```python
from build123d import *

# Parameters (mm, degrees)
CROQUIS1_W              = 15
CROQUIS1_H              = 12
SALIENTE_EXTRUIR1_DEPTH = 2
CORTAR_EXTRUIR1_REACH   = 11.811
CROQUIS2_R              = 2
CROQUIS3_W              = 33
CROQUIS3_H              = 17
SALIENTE_EXTRUIR2_DEPTH = 2
CORTAR_EXTRUIR3_REACH   = 26.192
CROQUIS5_W              = 8
CROQUIS5_H              = 3
CORTAR_EXTRUIR4_REACH   = 27.244
CROQUIS6_R              = 2
REDONDEO1_R             = 3
REDONDEO2_R             = 3


with BuildPart() as part:
    # Croquis1 → Saliente-Extruir1 (new body)
    with BuildSketch(Plane(origin=(0, 0, 0), x_dir=(1, 0, 0), z_dir=(0, 1, 0))):
        Rectangle(CROQUIS1_W, CROQUIS1_H)
    extrude(amount=SALIENTE_EXTRUIR1_DEPTH)

    # Croquis2 → Cortar-Extruir1 (cut, up to next)
    with BuildSketch(Plane(origin=(0, 2, 0), x_dir=(1, 0, 0), z_dir=(0, 1, 0)), mode=Mode.PRIVATE) as cortar_extruir1_sk1:
        with Locations(Location((-4.5, -3, 0), (0, 0, 270))):
            Circle(CROQUIS2_R)
    cortar_extruir1_tool1 = extrude(cortar_extruir1_sk1.sketch, amount=-CORTAR_EXTRUIR1_REACH, mode=Mode.PRIVATE) & part.part
    # Croquis2 → Cortar-Extruir1 (cut, up to next)
    with BuildSketch(Plane(origin=(0, 2, 0), x_dir=(1, 0, 0), z_dir=(0, 1, 0)), mode=Mode.PRIVATE) as cortar_extruir1_sk2:
        with Locations(Location((4.5, -3, 0), (0, 0, 270))):
            Circle(CROQUIS2_R)
    cortar_extruir1_tool2 = extrude(cortar_extruir1_sk2.sketch, amount=-CORTAR_EXTRUIR1_REACH, mode=Mode.PRIVATE) & part.part
    add(cortar_extruir1_tool1.solids().sort_by_distance((-4.5, 2, 3))[0], mode=Mode.SUBTRACT)
    add(cortar_extruir1_tool2.solids().sort_by_distance((4.5, 2, 3))[0], mode=Mode.SUBTRACT)

    # Croquis3 → Saliente-Extruir2 (add)
    with BuildSketch(Plane(origin=(0, 0, -6), x_dir=(-1, 0, 0), z_dir=(0, 0, -1))):
        with Locations((0, 4.5)):
            Rectangle(CROQUIS3_W, CROQUIS3_H)
    extrude(amount=SALIENTE_EXTRUIR2_DEPTH)

    # Croquis5 → Cortar-Extruir3 (cut, up to next)
    with BuildSketch(Plane.XY.offset(-6), mode=Mode.PRIVATE) as cortar_extruir3_sk1:
        with Locations((0, 4.5)):
            Rectangle(CROQUIS5_W, CROQUIS5_H)
    cortar_extruir3_tool1 = extrude(cortar_extruir3_sk1.sketch, amount=-CORTAR_EXTRUIR3_REACH, mode=Mode.PRIVATE) & part.part
    add(cortar_extruir3_tool1.solids().sort_by_distance((0, 4.5, -6))[0], mode=Mode.SUBTRACT)

    # Croquis6 → Cortar-Extruir4 (cut, up to next)
    with BuildSketch(Plane(origin=(0, 0, -8), x_dir=(-1, 0, 0), z_dir=(0, 0, -1)), mode=Mode.PRIVATE) as cortar_extruir4_sk1:
        with Locations((-11.5, 4.5)):
            Circle(CROQUIS6_R)
    cortar_extruir4_tool1 = extrude(cortar_extruir4_sk1.sketch, amount=-CORTAR_EXTRUIR4_REACH, mode=Mode.PRIVATE) & part.part
    # Croquis6 → Cortar-Extruir4 (cut, up to next)
    with BuildSketch(Plane(origin=(0, 0, -8), x_dir=(-1, 0, 0), z_dir=(0, 0, -1)), mode=Mode.PRIVATE) as cortar_extruir4_sk2:
        with Locations((11.5, 4.5)):
            Circle(CROQUIS6_R)
    cortar_extruir4_tool2 = extrude(cortar_extruir4_sk2.sketch, amount=-CORTAR_EXTRUIR4_REACH, mode=Mode.PRIVATE) & part.part
    add(cortar_extruir4_tool1.solids().sort_by_distance((11.5, 4.5, -8))[0], mode=Mode.SUBTRACT)
    add(cortar_extruir4_tool2.solids().sort_by_distance((-11.5, 4.5, -8))[0], mode=Mode.SUBTRACT)

    # Redondeo1
    redondeo1_edges = [part.edges().sort_by_distance(p)[0] for p in [
        (16.5, 13, -7),
        (16.5, -4, -7),
        (-16.5, -4, -7),
        (-16.5, 13, -7),
    ]]
    fillet(redondeo1_edges, radius=REDONDEO1_R)

    # Redondeo2
    redondeo2_edges = [part.edges().sort_by_distance(p)[0] for p in [
        (7.5, 1, 6),
        (-7.5, 1, 6),
    ]]
    fillet(redondeo2_edges, radius=REDONDEO2_R)


solid = part.part
```
Here's how the part is built. I have some questions about the finished solid (model axes, mm). A direction names the side the tool comes from. Coordinates: 2 decimals unless noted, no trailing zeros. Write each loop counter-clockwise with the first axis right and the second up, starting at its lowest first coordinate (ties: lowest second). Pieces come first, ordered by that corner, then holes. Notation, with made-up numbers: (-17.75, 13) -> (5.25, 13) arc R22 cw to (5.25, 45) -> close; hole circle Ø4 at (46, 31). An arc over 180 degrees is marked (long way). Use a Markdown table: item, result. Add a question column.
(1) If we section it at A-A, the plane y = 4.5: Write out the boundary of the cut face in (x, z), and give its area (3 significant figures).
(2) If we section it at C-C, the plane x = 3: Write out the boundary of the cut face in (y, z), and give its area (3 significant figures).
(3) We'd pull the mould along X, two halves only. Please class faces 5 (the flat face through (0, 3, -7)), 6 (the flat face through (0, 13, -7)), 7 (the cylindrical face through (-6.452, 1.014, 2.566)), 8 (the flat face through (-16.5, 4, -7)): +X half, -X half, draft (parallel to the pull), parting line (faces both ways), or undercut.
(4) If we section it at D-D, the plane x = -8: Write out the boundary of the cut face in (y, z), and give its area (3 significant figures).
(5) I'm going to push flat-ended pins straight in: P1, Ø3, axis at x = 11.5, y = 4.5, coming from the +Z side; P2, Ø5, axis at x = -5.5, z = 1.5, coming from the +Y side; P3, Ø1.6, axis at y = 0.5, z = -3, coming from the +X side; P4, Ø8, axis at y = 4.5, z = 3.5, coming from the -X side. Where does each tip first touch, or does it pass through?
(6) If we section it at B-B, the plane x = -11.5: Write out the boundary of the cut face in (y, z), and give its area (3 significant figures).
(7) Please list where these lines run through material, in increasing order: line 1 (X direction, y = 3.75, z = -6.5); line 2 (X direction, y = 1, z = 3.25); line 3 (Y direction, x = -11.5, z = -7.35).
(8) For faces 1 (the flat face through (0, 2, 0)), 2 (the flat face through (4, 4, -7)), 3 (the flat face through (0, 0, 0)), 4 (the flat face through (16.5, 4, -7)), which set-ups out of +Z, -Z, +X, -X, +Y, -Y let a thin tool reach every point of the face, with its end or its side?
Outcome:
| question | item | result |
|---|---|---|
| 1 | outline | (-16.5, -8) -> (-13.5, -8) -> (-13.5, -6) -> (-16.5, -6) -> close; (-9.5, -8) -> (-4, -8) -> (-4, -6) -> (-9.5, -6) -> close; (4, -8) -> (9.5, -8) -> (9.5, -6) -> (4, -6) -> close; (13.5, -8) -> (16.5, -8) -> (16.5, -6) -> (13.5, -6) -> close |
| 1 | area | 34.0 mm^2 |
| 2 | outline | (-4, -8) -> (3, -8) -> (3, -6) -> (2, -6) -> (2, 1.68) -> (0, 1.68) -> (0, -6) -> (-4, -6) -> close; (0, 4.32) -> (2, 4.32) -> (2, 6) -> (0, 6) -> close; (6, -8) -> (13, -8) -> (13, -6) -> (6, -6) -> close |
| 2 | area | 46.7 mm^2 |
| 3 | face 5 | undercut |
| 3 | face 6 | draft |
| 3 | face 7 | undercut |
| 3 | face 8 | -X half |
| 4 | outline | (-4, -8) -> (13, -8) -> (13, -6) -> (-4, -6) -> close |
| 4 | area | 34.0 mm^2 |
| 5 | P1 | passes through |
| 5 | P2 | stops at y = 2 |
| 5 | P3 | stops at x = 7.5 |
| 5 | P4 | stops at x = -7.5 |
| 6 | outline | (-4, -8) -> (2.5, -8) -> (2.5, -6) -> (-4, -6) -> close; (6.5, -8) -> (13, -8) -> (13, -6) -> (6.5, -6) -> close |
| 6 | area | 26.0 mm^2 |
| 7 | line 1 | x = -16.5 to -13.35, -9.65 to -4, 4 to 9.65, 13.35 to 16.5 |
| 7 | line 2 | x = -7.49 to -6.48, -2.52 to 2.52, 6.48 to 7.49 |
| 7 | line 3 | y = -4 to 2.5, 6.5 to 13 |
| 8 | face 1 | +Z, +X, -X, +Y |
| 8 | face 2 | +Z, -Z |
| 8 | face 3 | +Z, +X, -X, -Y |
| 8 | face 4 | +Z, -Z, +X, +Y, -Y |
